Design review of the part built by this model. Coordinates are the model's own, in mm. Face numbers are marked on the shaded views. A direction names the side the tool comes from. Coordinates: 2 decimals unless noted, no trailing zeros. Write each loop counter-clockwise with the first axis right and the second up, starting at its lowest first coordinate (ties: lowest second). Pieces come first, ordered by that corner, then holes. Notation, with made-up numbers: M 12.5,49.25 L 50.5,49.25 A20 cw 50.5,88.25 Z; hole C 10.25,-20 d1. An arc over 180 degrees is marked long. Return JSON: item names as keys, results as strings. Group by question number.
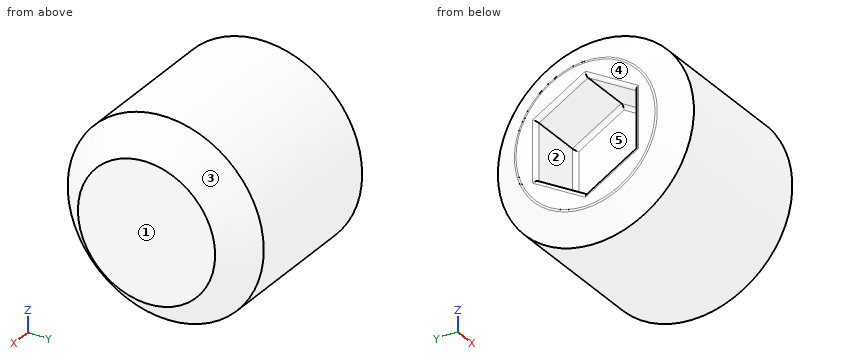
```python
from build123d import *

# Parameters (mm, degrees)
SKETCH_1_W          = 5
SKETCH_1_H          = 2.5
CUT_EXTRUDE_1_DEPTH = 1.5
CHAMFER_1_SIZE      = 0.75
CHAMFER_2_SIZE      = 0.7
CHAMFER_2_SIZE2     = 0.404145188
FILLET_1_R          = 0.1


with BuildPart() as part:
    # Эскиз1 → Повернуть1 (revolve)
    with BuildSketch(Plane(origin=(0, 0, 0), x_dir=(-1, 0, 0), z_dir=(0, 0, -1))):
        with Locations((-2.5, 1.25)):
            Rectangle(SKETCH_1_W, SKETCH_1_H)
    revolve(axis=Axis((5, 0, 0), (-1, 0, 0)))

    # Эскиз2 → Вырез-Вытянуть1 (cut)
    with BuildSketch(Plane.ZY):
        Polygon((0.721687836, -1.25), (1.443375673, 0), (0.721687836, 1.25), (-0.721687836, 1.25), (-1.443375673, 0), (-0.721687836, -1.25), align=None)
    extrude(amount=-CUT_EXTRUDE_1_DEPTH, mode=Mode.SUBTRACT)

    # Фаска1
    chamfer_1_edges = [part.edges().sort_by_distance(p)[0] for p in [
        (5, -2.5, 0),
    ]]
    chamfer(chamfer_1_edges, length=CHAMFER_1_SIZE)

    # Фаска2
    chamfer_2_edges = [part.edges().sort_by_distance(p)[0] for p in [
        (0, -2.5, 0),
    ]]
    chamfer_2_side = [part.faces().sort_by_distance(p)[0] for p in [
        (0, -2.429289322, 0),
    ]]
    chamfer(chamfer_2_edges, length=CHAMFER_2_SIZE, length2=CHAMFER_2_SIZE2, reference=chamfer_2_side[0])

    # Скругление1
    fillet_1_edges = [part.edges().sort_by_distance(p)[0] for p in [
        (1.5, -1.25, 0),
        (1.5, -0.625, -1.082531755),
        (1.5, 0.625, -1.082531755),
        (1.5, 1.25, 0),
        (1.5, 0.625, 1.082531755),
        (1.5, -0.625, 1.082531755),
        (0, -1.25, 0),
        (0, -0.625, 1.082531755),
        (0, 0.625, 1.082531755),
        (0, 1.25, 0),
        (0, 0.625, -1.082531755),
        (0, -0.625, -1.082531755),
        (0, -1.8, 0),
    ]]
    fillet(fillet_1_edges, radius=FILLET_1_R)


solid = part.part
```
Item 1: The part is to be moulded in two halves that separate along Z. For the marked faces 1, 2 and 3, say which applies: pulls with the +Z half, pulls with the -Z half, needs draft (parallel to the pull), parting line crosses it, or undercut.
Item 2: Add section C-C (x = 3.7). Write out the cut boundary in (y, z).
Item 3: Machinability: for the marked faces 4 and 5, which of the approach directions +Z, -Z, +X, -X, +Y, -Y give a long, thin tool a straight path to every point of the face, cutting with its end or side? Answer none if there is none.
Item 4: Add section B-B (x = 4.6). Write out the cut boundary in (y, z).
Item 5: Add section A-A (z = 0). Write out the cut boundary in (x, y).
Item 6: For line 1 (X direction, y = 0, z = 1); line 2 (Y direction, x = 0.5, z = -0.65); line 3 (Z direction, x = 0.55, y = 1.9), list the stretches that pass through material, from the lowest coordinate up.
Geometry check:
{
 "1": {"face 1": "needs draft", "face 2": "undercut", "face 3": "parting line crosses it"},
 "2": {"outline": "C 0,0 d5"},
 "3": {"face 4": "+Z, -Z, -X, +Y, -Y", "face 5": "-X"},
 "4": {"outline": "C 0,0 d4.3"},
 "5": {"outline": "M 0,-1.77 A0.1 ccw 0.01,-1.82 L 0.4,-2.5 L 4.25,-2.5 L 5,-1.75 L 5,1.75 L 4.25,2.5 L 0.4,2.5 L 0.01,1.82 A0.1 ccw 0,1.77 L 0,1.35 A0.1 ccw 0.1,1.25 L 1.4,1.25 A0.1 cw 1.5,1.15 L 1.5,-1.15 A0.1 cw 1.4,-1.25 L 0.1,-1.25 A0.1 ccw 0,-1.35 Z"},
 "6": {"line 1": "1.5 to 5", "line 2": "-2.41 to -1.25, 1.25 to 2.41", "line 3": "-1.62 to 1.62"}
}
